```python
from build123d import *

# Parameters (mm, degrees)
F0_W     = 139.181651175
F0_H     = 178.9838671684
F1_DEPTH = 76.2
F2_W     = 122.5202530622
F2_H     = 60.2431138977
F3_DEPTH = 172.72
F4_W     = 131.1423294246
F4_H     = 60.5337903835
F5_DEPTH = 25.4
F7_DEPTH = 25.4
F8_W     = 122.8211522102
F8_H     = 166.64852947
F9_DEPTH = 14.224


with BuildPart() as f1:
    # F0 (on Top) → F1 (new body)
    with BuildSketch(Plane.XY):
        with Locations((-2.3464225233, 20.7241773605)):
            Rectangle(F0_W, F0_H)
    extrude(amount=F1_DEPTH)

    # F2 (on face) → F3 (cut)
    with BuildSketch(Plane.XZ.offset(68.7677562237)):
        with Locations((-3.7967562675, 34.5050995238)):
            Rectangle(F2_W, F2_H)
    extrude(amount=-F3_DEPTH, mode=Mode.SUBTRACT)

    # F4 (on face) → F5 (cut)
    with BuildSketch(Plane(origin=(-71.9372481108, 0, 0), x_dir=(0, -1, 0), z_dir=(-1, 0, 0))):
        with Locations((-2.1996553987, 36.2956381869)):
            Rectangle(F4_W, F4_H)
    extrude(amount=-F5_DEPTH, mode=Mode.SUBTRACT)

    # F6 (on face) → F7 (join)
    with BuildSketch(Plane.XY.offset(4.3835425749)):
        Polygon((57.4633702636, 103.9522437763), (-46.4984178543, 103.9522437763), (-46.4984178543, 83.275783987), (38.8480201364, 83.275783987), (38.8480201364, 16.3331480634), (57.4633702636, 16.3331480634), align=None)
    extrude(amount=F7_DEPTH)

    # F8 (on face) → F9 (cut)
    with BuildSketch(Plane.XY.offset(76.2)):
        with Locations((-4.2247846723, 18.8339464366)):
            Rectangle(F8_W, F8_H)
    extrude(amount=-F9_DEPTH, mode=Mode.SUBTRACT)


solid = f1.part
```
For this review, take the finished solid that the model builds, in its own axes (mm). A direction names the side the tool comes from. Coordinates: 2 decimals unless noted, no trailing zeros. Loops run counter-clockwise (first coordinate to the right, second up) from the corner with the lowest first, then second, coordinate; pieces in that order, holes last.
1. Insertion check: P1, Ø2, axis at x = -12, z = 20, coming from the -Y side; P2, Ø6, axis at y = -12, z = 39.5, coming from the -X side; P3, Ø9.5, axis at x = 51, z = 12.5, coming from the -Y side; P4, Ø1.9, axis at x = -68.5, y = -28.5, coming from the -Z side. Each pin has a flat end and moves straight along its axis. Give the tip position at first contact, or say it passes through.
2. Add section A-A, the plane z = 70.5. Give the boundary of the cut face in (x, y).
3. For line 1 (X direction, y = 74, z = 40); line 2 (Y direction, x = 29.5, z = 66.5); line 3 (X direction, y = -4, z = 68), list the stretches that pass through material, from the lowest coordinate up.
4. For faces 4 (the flat face through (-4, 83.276, 17)), 5 (the flat face through (-5, 102.158, 71)), 6 (the flat face through (-69, 3, 6.029)), list the 3-axis set-ups (+Z, -Z, +X, -X, +Y, -Y) from which the entire face can be reached by the end or side of a thin tool; tool diameter is ignored.
5. Add section D-D, the plane z = 40. Give the boundary of the cut face in (x, y), then the cut area to 3 significant figures.
6. Add section B-B, the plane x = -27. Give the boundary of the cut face in (y, z).
7. Add section C-C, the plane y = 33. Give the boundary of the cut face in (x, z).
8. Mouldability with a two-part tool opening along Y and no side actions: class faces 1 (the flat face through (-3, 110.216, 38)), 2 (the flat face through (67.244, 19, 38)), 3 (the flat face through (-69, 67.771, 36)) as +Y half, -Y half, draft (parallel to the pull), parting line (faces both ways), or undercut.
Result:
1. P1: stops at y = 83.28
1. P2: stops at x = 57.46
1. P3: stops at y = 16.33
1. P4: stops at z = 0
2. outline: (-71.94, -68.77) - (67.24, -68.77) - (67.24, 110.22) - (-71.94, 110.22) - close; hole (-65.64, -64.49) - (57.19, -64.49) - (57.19, 102.16) - (-65.64, 102.16) - close
3. line 1: x = -71.94 to -65.06, 57.46 to 67.24
3. line 2: y = -68.77 to -64.49, 102.16 to 110.22
3. line 3: x = -71.94 to -65.64, 57.19 to 67.24
4. face 4: +Z, -Y
4. face 5: +Z
4. face 6: -X
5. outline: (-71.94, -68.77) - (-65.06, -68.77) - (-65.06, -63.37) - (-71.94, -63.37) - close; (-71.94, 67.77) - (-65.06, 67.77) - (-65.06, 103.95) - (57.46, 103.95) - (57.46, -68.77) - (67.24, -68.77) - (67.24, 110.22) - (-71.94, 110.22) - close
5. area: 2,850 mm2
6. outline: (-68.77, 0) - (110.22, 0) - (110.22, 76.2) - (102.16, 76.2) - (102.16, 64.63) - (103.95, 64.63) - (103.95, 29.78) - (83.28, 29.78) - (83.28, 4.38) - (-68.77, 4.38) - close; (-68.77, 64.63) - (-64.49, 64.63) - (-64.49, 76.2) - (-68.77, 76.2) - close
7. outline: (-71.94, 0) - (67.24, 0) - (67.24, 76.2) - (57.19, 76.2) - (57.19, 64.63) - (57.46, 64.63) - (57.46, 29.78) - (38.85, 29.78) - (38.85, 4.38) - (-65.06, 4.38) - (-65.06, 6.03) - (-71.94, 6.03) - close; (-71.94, 66.56) - (-65.64, 66.56) - (-65.64, 76.2) - (-71.94, 76.2) - close
8. face 1: +Y half
8. face 2: draft
8. face 3: undercut
